Work out the finished part from the listing and answer in its coordinate system (mm). A direction names the side the tool comes from. Round coordinates to 2 decimals unless told otherwise and drop trailing zeros. Loops run counter-clockwise (first coordinate to the right, second up) from the corner with the lowest first, then second, coordinate; pieces in that order, holes last.
```python
from build123d import *

# Parameters (mm, degrees)
SKETCH_1_R      = 2.5
SKETCH_1_R_2    = 13.5
SKETCH_1_R_3    = 5
EXTRUDE_1_DEPTH = 3
SKETCH_1_3_R    = 13.5
SKETCH_1_3_R_2  = 5
EXTRUDE_2_DEPTH = 8.5
SKETCH_1_4_R    = 5
SKETCH_1_4_R_2  = 4
EXTRUDE_3_DEPTH = 13


with BuildPart() as part:
    # Sketch 1 → Extrude 1 (new body)
    # profile 1 of 3: a face of its own
    with BuildSketch(Plane.XY):
        with BuildLine():
            Line((-24, 2.5), (-24, -2.5))
            Line((-24, -2.5), (-6.352941176, -11.911764706))
            ThreePointArc((-6.352941176, -11.911764706), (-13.5, 0), (-6.352941176, 11.911764706))
            Line((-6.352941176, 11.911764706), (-24, 2.5))
        make_face()
        with Locations((-18, 0)):
            Circle(SKETCH_1_R, mode=Mode.SUBTRACT)
    # profile 2 of 3: a face of its own
    with BuildSketch(Plane.XY):
        Circle(SKETCH_1_R_2)
        Circle(SKETCH_1_R_3, mode=Mode.SUBTRACT)
    # profile 3 of 3: a face of its own
    with BuildSketch(Plane.XY):
        with BuildLine():
            ThreePointArc((13.5, 0), (11.576154497, -6.945692698), (6.352941176, -11.911764706))
            Line((6.352941176, -11.911764706), (24, -2.5))
            Line((24, -2.5), (24, 2.5))
            Line((24, 2.5), (6.352941176, 11.911764706))
            ThreePointArc((6.352941176, 11.911764706), (11.576154497, 6.945692698), (13.5, 0))
        make_face()
        with Locations((18, 0)):
            Circle(SKETCH_1_R, mode=Mode.SUBTRACT)
    extrude(amount=EXTRUDE_1_DEPTH)

    # Sketch 1_3 → Extrude 2 (add)
    with BuildSketch(Plane.XY):
        with Locations(Location((0, 0, 0), (0, 0, 118.072486936))):
            Circle(SKETCH_1_3_R)
        Circle(SKETCH_1_3_R_2, mode=Mode.SUBTRACT)
    extrude(amount=EXTRUDE_2_DEPTH)

    # Sketch 1_4 → Extrude 3 (add)
    with BuildSketch(Plane.XY):
        with Locations(Location((0, 0, 0), (0, 0, 180))):
            Circle(SKETCH_1_4_R)
        with Locations(Location((0, 0, 0), (0, 0, 180))):
            Circle(SKETCH_1_4_R_2, mode=Mode.SUBTRACT)
    extrude(amount=EXTRUDE_3_DEPTH)


solid = part.part
```
1. Find section C-C (z = 10.5). Write down the section's boundary in (x, y), then the cut area to 3 significant figures.
Answer key:
outline: circle Ø10 at (0, 0); hole circle Ø8 at (0, 0)
area: 28.3 mm2
2. Determine the mould class of faces 3 (the face through (24, 0, 1)), 4 (the face through (0.867, 3.905, 6.409)), 5 (the face through (-15.3, -7.14, 1.48)), 6 (the face through (-20.5, 0.1, 1.5)) for opening direction Y: +Y half, -Y half, draft (parallel to the pull), parting line (faces both ways), or undercut.
Answer key:
face 3: draft
face 4: undercut
face 5: -Y half
face 6: undercut
3. Given pin 1 (6.5 mm diameter, centred on x = -18, y = 0, fed in from +Z); pin 2 (10 mm diameter, centred on x = -17.5, y = -2, fed in from +Z); pin 3 (6 mm diameter, centred on x = -8, z = 4, fed in from -Y); pin 4 (4 mm diameter, centred on x = 18, y = 0, fed in from -Z), each flat-ended and moving along its own axis, determine where each tip first touches the part or whether it passes through.
Answer key:
pin 1: stops at z = 3
pin 2: stops at z = 8.5
pin 3: stops at y = -12.54
pin 4: passes through
4. Find section A-A (x = 18). Write down the section's boundary in (y, z).
Answer key:
outline: (-5.7, 0) - (-2.5, 0) - (-2.5, 3) - (-5.7, 3) - close; (2.5, 0) - (5.7, 0) - (5.7, 3) - (2.5, 3) - close
5. Which of the six approach directions +Z, -Z, +X, -X, +Y, -Y give full straight-line access (tool end or side, diameter ignored) to faces 1 (the face through (5, 0, 11)), 2 (the face through (15.053, -7.272, 1.479))?
Answer key:
face 1: +Z
face 2: +Z, -Z, +X, -Y
6. Consider probe 1 along Y at (x, z) = (0, 7.25); probe 2 along Z at (x, y) = (-9.5, 0.75); probe 3 along Z at (x, y) = (22, -2). Determine where each line is inside the solid, lowest interval first.
Answer key:
probe 1: y = -13.5 to -4, 4 to 13.5
probe 2: z = 0 to 8.5
probe 3: z = 0 to 3
7. Find section D-D (x = 0). Write down the section's boundary in (y, z).
Answer key:
outline: (-13.5, 0) - (-4, 0) - (-4, 13) - (-5, 13) - (-5, 8.5) - (-13.5, 8.5) - close; (4, 0) - (13.5, 0) - (13.5, 8.5) - (5, 8.5) - (5, 13) - (4, 13) - close
8. Find section B-B (y = 0). Write down the section's boundary in (x, z), then the cut area to 4 significant figures.
Answer key:
outline: (-24, 0) - (-20.5, 0) - (-20.5, 3) - (-24, 3) - close; (-15.5, 0) - (-4, 0) - (-4, 13) - (-5, 13) - (-5, 8.5) - (-13.5, 8.5) - (-13.5, 3) - (-15.5, 3) - close; (4, 0) - (15.5, 0) - (15.5, 3) - (13.5, 3) - (13.5, 8.5) - (5, 8.5) - (5, 13) - (4, 13) - close; (20.5, 0) - (24, 0) - (24, 3) - (20.5, 3) - close
area: 203.5 mm2
